Input: part model. Units: mm. Frame: model coordinates. Face numbers are marked on the shaded views. A direction names the side the tool comes from. Give positions to 0.01 mm unless a question says otherwise; leave off trailing zeros. Order: outer loops, then holes, each group sorted by start corner. A loop starts at its lowest first (then second) coordinate and runs counter-clockwise, first axis right, second up.
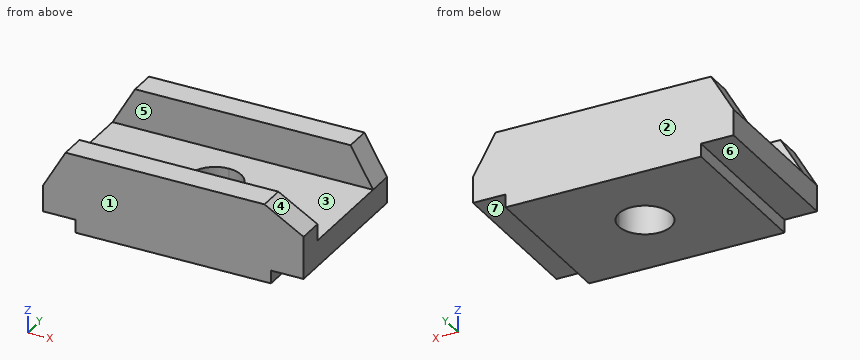
```python
from build123d import *

# Parameters (mm, degrees)
F1_DEPTH    = 76.2
F2_W        = 127
F2_H        = 50.8
F3_DEPTH    = 19.05
F4_C1_SIZE2 = 10.9985226281
F4_C1_SIZE  = 19.05
F4_C2_SIZE2 = 10.9985226281
F4_C2_SIZE  = 19.05
F4_C3_SIZE2 = 19.05
F4_C3_SIZE  = 10.9985226281
F4_C4_SIZE2 = 19.05
F4_C4_SIZE  = 10.9985226281
F6_DEPTH    = 56.642


with BuildPart() as f1:
    # F0 (on Front) → F1 (new body)
    with BuildSketch(Plane.XZ):
        Polygon((15.875, 6.35), (15.875, 0), (111.125, 0), (111.125, 6.35), (127, 6.35), (127, 19.05), (127, 38.1), (0, 38.1), (0, 19.05), (0, 6.35), align=None)
    extrude(amount=F1_DEPTH)

    # F2 (on face) → F3 (cut)
    with BuildSketch(Plane.XY.offset(38.1)):
        with Locations((63.5, -38.1)):
            Rectangle(F2_W, F2_H)
    extrude(amount=-F3_DEPTH, mode=Mode.SUBTRACT)

    # F4: chamfer of 19.05 x 10.9985226281 on 4 edges, made by hand

    # F4_c1
    f4_c1_edges = [f1.edges().sort_by_distance(p)[0] for p in [
        (0, -69.85, 38.1),
    ]]
    f4_c1_side = f1.faces().sort_by_distance((0, -69.85, 37.8800295474))[0]
    chamfer(f4_c1_edges, length=F4_C1_SIZE, length2=F4_C1_SIZE2, reference=f4_c1_side)

    # F4_c2
    f4_c2_edges = [f1.edges().sort_by_distance(p)[0] for p in [
        (0, -6.35, 38.1),
    ]]
    f4_c2_side = f1.faces().sort_by_distance((0, -6.35, 37.8800295474))[0]
    chamfer(f4_c2_edges, length=F4_C2_SIZE, length2=F4_C2_SIZE2, reference=f4_c2_side)

    # F4_c3
    f4_c3_edges = [f1.edges().sort_by_distance(p)[0] for p in [
        (127, -6.35, 38.1),
    ]]
    f4_c3_side = f1.faces().sort_by_distance((126.7800295474, -6.35, 38.1))[0]
    chamfer(f4_c3_edges, length=F4_C3_SIZE, length2=F4_C3_SIZE2, reference=f4_c3_side)

    # F4_c4
    f4_c4_edges = [f1.edges().sort_by_distance(p)[0] for p in [
        (127, -69.85, 38.1),
    ]]
    f4_c4_side = f1.faces().sort_by_distance((127, -69.85, 37.8800295474))[0]
    chamfer(f4_c4_edges, length=F4_C4_SIZE, length2=F4_C4_SIZE2, reference=f4_c4_side)

    # F5 (on face) → F6 (cut)
    with BuildSketch(Plane.XY.offset(19.05)):
        with BuildLine():
            ThreePointArc((76.2, -38.1), (72.4802561211, -29.1197438789), (63.5, -25.4))
            ThreePointArc((63.5, -25.4), (54.5197438789, -47.0802561211), (76.2, -38.1))
        make_face()
    extrude(amount=-F6_DEPTH, mode=Mode.SUBTRACT)


solid = f1.part
```
1) Reachability of the marked faces 4, 5, 6 and 7 from +Z, -Z, +X, -X, +Y, -Y: full face, straight path, thin tool, end or side. Return the list, or none.
2) First-contact query: P1, Ø3, axis at y = -21.5, z = 2, coming from the -X side (3 decimals); P2, Ø5, axis at x = 111, y = -26, coming from the -Z side; P3, Ø5, axis at x = 122, y = -21.5, coming from the -Z side; P4, Ø5, axis at y = -28, z = 2, coming from the +X side (3 decimals). Flat tips, straight axial feed; report the tip coordinate or a pass-through.
3) Cut plane B-B (x = 78). Return the cut outline in (y, z).
4) Cut plane D-D (x = 112.5). Return the cut outline in (y, z).
5) Line query: probe 1 along X at (y, z) = (-38, 10); probe 2 along Y at (x, z) = (63.5, 5.5); probe 3 along Y at (x, z) = (108, 26). Output: solid intervals per line, ascending.
6) Pull-direction query (Y, two-part tool) for the marked faces 1, 2 and 3; classes: pulls with the +Y half, pulls with the -Y half, needs draft (parallel to the pull), parting line crosses it, or undercut.
7) Cut plane A-A (y = -27.5). Return the cut outline in (x, z) (3 decimals).
8) Cut plane C-C (y = -44). Return the cut outline in (x, z) (3 decimals), then the cut area to 3 significant figures.
Geometry says:
1. face 4: +Z, +X, -Y
1. face 5: +Z, +X, -X
1. face 6: -Z, -X, +Y, -Y
1. face 7: -Z, +X, +Y, -Y
2. P1: stops at x = 15.875
2. P2: stops at z = 0
2. P3: stops at z = 6.35
2. P4: stops at x = 111.125
3. outline: (-76.2, 0) - (0, 0) - (0, 38.1) - (-12.7, 38.1) - (-12.7, 19.05) - (-63.5, 19.05) - (-63.5, 38.1) - (-76.2, 38.1) - close
4. outline: (-76.2, 6.35) - (0, 6.35) - (0, 38.1) - (-12.7, 38.1) - (-12.7, 19.05) - (-63.5, 19.05) - (-63.5, 35.47) - (-76.2, 35.47) - close
5. probe 1: x = 0 to 50.8, 76.2 to 127
5. probe 2: y = -76.2 to -50.8, -25.4 to 0
5. probe 3: y = -76.2 to -63.5, -12.7 to 0
6. face 1: pulls with the -Y half
6. face 2: pulls with the +Y half
6. face 3: undercut
7. outline: (0, 6.35) - (15.875, 6.35) - (15.875, 0) - (56.505, 0) - (56.505, 19.05) - (0, 19.05) - close; (70.495, 0) - (111.125, 0) - (111.125, 6.35) - (127, 6.35) - (127, 19.05) - (70.495, 19.05) - close
8. outline: (0, 6.35) - (15.875, 6.35) - (15.875, 0) - (52.254, 0) - (52.254, 19.05) - (0, 19.05) - close; (74.746, 0) - (111.125, 0) - (111.125, 6.35) - (127, 6.35) - (127, 19.05) - (74.746, 19.05) - close
8. area: 1,790 mm2
